Can you work these out from the model? Positions are in its coordinate system, mm. Face numbers are marked on the shaded views. A direction names the side the tool comes from. Give positions to 0.01 mm unless a question says otherwise; leave off trailing zeros. Write item = value, one per line.
Autodesk Fusion 360 part; units mm, degrees
sketch "Sketch1" plane through (0, 0, 0) normal (0, 1, 0) x (1, 0, 0)
  circle A0 centre (-10, 0) radius 6.25
  circle A1 centre (-10, 0) radius 9
  circle A2 centre (10, 0) radius 6.25
  circle A3 centre (10, 0) radius 9
  line L0 (-23, -18) -> (23, -18)
  line L1 (23, -18) -> (23, 3)
  line L2 (13, 13) -> (-13, 13)
  line L3 (-23, 3) -> (-23, -18)
  line L4 (-23, -13) -> (23, -13)
  arc A4 (23, 3) -> (13, 13) centre (13, 3) ccw
  arc A5 (-13, 13) -> (-23, 3) centre (-13, 3) ccw
  dimension "d1" = 12.5
  dimension "d2" = 12.5
  dimension "d3" = 18
  dimension "d4" = 18
  dimension "d5" = 10
  dimension "d6" = 10
  dimension "d7" = 13
  dimension "d9" = 13
  dimension "d10" = 10
  dimension "d11" = 13
  dimension "d12" = 10
  dimension "d13" = 13
  dimension "d14" = 5
extrude "Extrude1" add sketch "Sketch1" against normal blind 2 contours A1 | A3 | L0 L1 L3 L4 | L1 L2 L3 L4 A4 A5
extrude "Extrude2" add sketch "Sketch1" along normal blind 15 contours L0 L1 L3 L4
sketch "Sketch2" plane through (0, 0, 13) normal (0, 0, -1) x (1, 0, 0)
  line L0 (23, 0) -> (-23, 0)
  line L1 (-23, 0) -> (-23, -15)
  line L2 (-23, -15) -> (23, -15)
  line L3 (23, -15) -> (23, 0)
  circle A0 centre (13, -7.5) radius 2.5
  circle A1 centre (-13, -7.5) radius 2.5
  circle A2 centre (-13, -7.5) radius 5
  circle A3 centre (13, -7.5) radius 5
  dimension "d19" = 5
  dimension "d20" = 5
  dimension "d21" = 10
  dimension "d22" = 10
  dimension "d23" = 7.5
  dimension "d24" = 7.5
  dimension "d25" = 10
  dimension "d26" = 10
extrude "Extrude3" cut sketch "Sketch2" against normal up to surface (5 mm away) contours A0 | A1
extrude "Extrude4" cut sketch "Sketch2" against normal up to surface (3 mm away) contours A2 | A3
chamfer "Chamfer1" distance 2.5 angle 45 2 edges at (8.3384, 9.3081, 16) (-17.6616, 9.3081, 16)
fillet "Fillet1" radius 10 2 edges at (23, 15, 15.5) (-23, 15, 15.5)
fillet "Fillet2" radius 3 1 edges at (0, 0, 13)
fillet "Fillet3" radius 1 17 edges at (-23, -2, 7.5) (-20.0711, -2, -10.0711) (0, -2, -13) (20.0711, -2, -10.0711) (23, -2, 7.5) (0, 15, 13) (-20.0711, 12.0711, 13) (-23, 4, 13) (-23, 0.8787, 12.1213) (-23, 0, 3.5) (-20.0711, 0, -10.0711) (0, 0, -13) (20.0711, 0, -10.0711) (23, 0, 3.5) (23, 0.8787, 12.1213) (23, 4, 13) (20.0711, 12.0711, 13)
equation "d1 = d2"
equation "d4 = d3"
equation "d9 = d7"
equation "d11 = d7"
equation "d13 = d7"
equation "d20 = d19"
equation "d22 = d21"
equation "d24 = d23"
equation "d26 = d25"
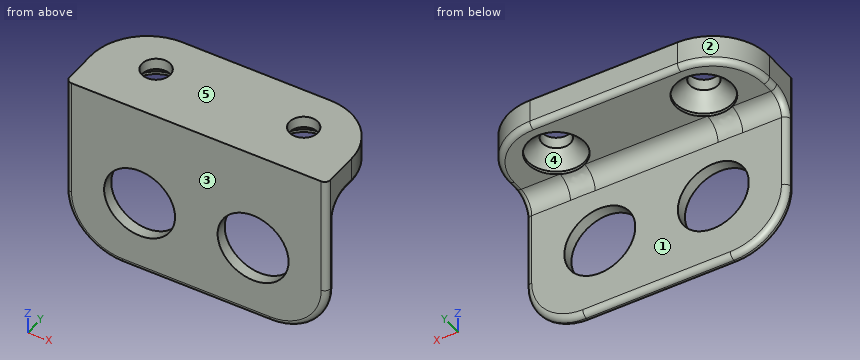
Q1. Imagine slicing it at A-A, the plane z = 0. Give the number of separate pieces and of enclosed holes in the cut face, then the cut area to 3 significant figures.
Output:
separate_pieces = 3
enclosed_holes = 0
area = 41.1 mm2
Q2. Which directions (+Z, -Z, +X, -X, +Y, -Y) give clear straight access to the entire face, cutting with the end or side of a thin tool? Please do the marked faces 1 and 2.
Output:
face_1 = -Z, +X, -X, +Y
face_2 = +Z, -Z, -X, +Y
Q3. I need wall thicknesses on L1, parallel to Z at x = 10, y = -0.9 (3 decimals); L2, parallel to Y at x = 13, z = 16; L3, parallel to X at y = 7.5, z = 13.45. Which ranges of each line are inside material? Lowest first, please.
Output:
L1 = -12.995 to -6.25, 6.25 to 18
L2 = -2 to 5, 10 to 15
L3 = -22.51 to -18, -8 to 8, 18 to 22.51
Q4. For pin 1 (5 mm diameter, centred on x = 7.5, y = 12, fed in from -Z); pin 2 (6 mm diameter, centred on x = 13, y = 7.5, fed in from -Z); pin 3 (4 mm diameter, centred on x = -14, y = 6.5, fed in from -Z), each with a flat end and sliding along its axis, tell me the tip position at first contact or that it passes through.
Output:
pin_1 = 13
pin_2 = 15.5
pin_3 = 15.09
Q5. We'd pull the mould along Y, two halves only. Please class the marked faces 3, 4 and 5: released by +Y, released by -Y, zero draft, split by the parting line, or undercut.
Output:
face_3 = released by -Y
face_4 = undercut
face_5 = zero draft
